Autodesk Inventor part; units mm, degrees
ref_plane "YZ Plane" through (0, 0, 0) normal (1, 0, 0) x (0, 1, 0)
ref_plane "XZ Plane" through (0, 0, 0) normal (0, 1, 0) x (-1, 0, 0)
ref_plane "XY Plane" through (0, 0, 0) normal (0, 0, 1) x (1, 0, 0)
sketch "Sketch1" plane through (0, 0, 0) normal (0, 1, 0) x (-1, 0, 0)
  circle A0 centre (0, 0) radius 35
  circle A1 centre (0, 0) radius 10.7
  line L0 (0, 0) -> (0, -48)
  line L1 (60, -48) -> (-60, -48)
  circle A2 centre (-60, -48) radius 50
  circle A3 centre (60, -48) radius 50
  circle A4 centre (0, 0) radius 20
  line L2 (73.5118, 0.1397) -> (5.4047, 19.2559)
  line L3 (-73.5118, 0.1397) -> (-5.4047, 19.2559)
  line L4 (0, 0) -> (0, -25)
  line L5 (24.4949, -25) -> (-24.4949, -25)
  circle A5 centre (0, 0) radius 27.5
  line L6 (0, 0) -> (-26.563, 7.1175)
  line L7 (0, 0) -> (27.5, 0) construction
  line L8 (0, 0) -> (-26.563, -7.1175)
  line L9 (0, 0) -> (26.563, 7.1175)
  line L10 (0, 0) -> (26.563, -7.1175)
  point P0 (33.0589, 11.494)
  point P1 (-33.0589, 11.494)
  dimension "d0" = 70
  dimension "d10" = 100
  dimension "d11" = 100
  dimension "d1" = 21.4
  dimension "d8" = 48
  dimension "d9" = 120
  dimension "d12" = 40
  dimension "d13" = 25
  dimension "d18" = 55
  dimension "d19" = 165
extrude "Extrusion1" add sketch "Sketch1" along normal blind 5 contours A0 A3 A5 L2 | A0 L5 A3 A5 | L3 A5 A2 A0 | A5 L9 A4 L2 | A5 A3 | A3 A5 L5 L0 A4 L10 | A2 A5 L5 A0 | L3 A4 L6 A5 | A4 L9 A1 L6 | A5 L10 A4 L9 | L5 A5 A3 | A5 L8 A4 L0 L5 A2 | A2 A5 | L6 A4 L8 A5 | A4 L10 A1 L9 | A4 L0 A1 L10 | A2 A5 L5 | L6 A1 L8 A4 | A4 L8 A1 L0
fillet "Fillet1" radius 10 4 edges at (33.0589, 2.5, 11.494) (-33.0589, 2.5, 11.494) (24.4949, 2.5, -25) (-24.4949, 2.5, -25)
sketch "Sketch3" plane through (0, 5, 0) normal (0, 1, 0) x (1, 0, 0)
  circle A0 centre (0, 0) radius 10.7
  circle A1 centre (0, 0) radius 15
  dimension "d15" = 30
extrude "Extrusion3" add sketch "Sketch3" along normal blind 30
hole "Hole1" at (26.563, 0, 7.1175) at (26.563, 0, -7.1175) at (-26.563, 0, 7.1175) at (-26.563, 0, -7.1175) direction (0, 1, 0) diameter 4 end through all
properties part number "SyringeHolder"
Source: CAD feature listing. Evaluate the final solid. Frame: model axes, mm. A direction names the side the tool comes from. Round coordinates to 2 decimals unless told otherwise and drop trailing zeros. Loops run counter-clockwise (first coordinate to the right, second up) from the corner with the lowest first, then second, coordinate; pieces in that order, holes last. Notation, with made-up numbers: M 50,64.5 L 80,64.5 A15 ccw 80,91.5 Z; hole C 53,-9 d10. An arc over 180 degrees is marked long. Use a Markdown table: item, result. Add a question column.
1. Contact query for flat-ended pins moving along their axis: P1, Ø4, axis at x = -7, y = 19.5, coming from the -Z side; P2, Ø3, axis at y = 20, z = 9.5, coming from the -X side; P3, Ø10, axis at x = -4.5, y = 31, coming from the +Z side. Output: stop coordinate, or through.
2. Reachability of faces 4 (the cylindrical face through (-14.985, 19.79, 0.66)), 5 (the cylindrical face through (-24.61, 2.54, 7.55)) from +Z, -Z, +X, -X, +Y, -Y: full face, straight path, thin tool, end or side. Return the list, or none.
3. Line query: line 1 (Z direction, x = 0, y = 27); line 2 (Y direction, x = 13.5, z = 8). Output: solid intervals per line, ascending.
4. Mould query, pull axis X, two halves, no side actions, for faces 1 (the cylindrical face through (28.515, 2.535, 7.551)), 2 (the flat face through (10, 35, 6)), 3 (the cylindrical face through (-32.35, 2.54, 9.95)). Classes: pulls with the +X half, pulls with the -X half, needs draft (parallel to the pull), parting line crosses it, or undercut.
5. Section query A-A on z = 0. Return the cut outline in (x, y).
6. Section query D-D on z = -16.5. Return the cut outline in (x, y), then the cut area to 3 significant figures.
7. Section query C-C on y = 26.5. Return the cut outline in (x, z).
8. Section query B-B on x = 0. Return the cut outline in (y, z), then the cut area to 3 significant figures.
Reported:
| question | item | result |
|---|---|---|
| 1 | P1 | stops at z = -14.14 |
| 1 | P2 | stops at x = -12.69 |
| 1 | P3 | stops at z = 15 |
| 2 | face 4 | +Y |
| 2 | face 5 | +Y, -Y |
| 3 | line 1 | z = -15 to -10.7, 10.7 to 15 |
| 3 | line 2 | y = 0 to 5 |
| 4 | face 1 | undercut |
| 4 | face 2 | needs draft |
| 4 | face 3 | pulls with the -X half |
| 5 | outline | M -35,0 L -10.7,0 L -10.7,35 L -15,35 L -15,5 L -35,5 Z; M 10.7,0 L 35,0 L 35,5 L 15,5 L 15,35 L 10.7,35 Z |
| 6 | outline | M -30.87,0 L 30.87,0 L 30.87,5 L -30.87,5 Z |
| 6 | area | 309 mm² |
| 7 | outline | C 0,0 d30; hole C 0,0 d21.4 |
| 8 | outline | M 0,-25 L 5,-25 L 5,-15 L 35,-15 L 35,-10.7 L 0,-10.7 Z; M 0,10.7 L 35,10.7 L 35,15 L 5,15 L 5,20 L 0,20 Z |
| 8 | area | 376 mm² |
